The model under review builds one solid part; all positions refer to its coordinate system, in mm. A direction names the side the tool comes from. Coordinates: 2 decimals unless noted, no trailing zeros. Order: outer loops, then holes, each group sorted by start corner. A loop starts at its lowest first (then second) coordinate and runs counter-clockwise, first axis right, second up. Notation, with made-up numbers: (-4.5, 81) -> (54.5, 81) arc R24 cw to (54.5, 105) -> close; hole circle Ø2 at (-17.5, -23). An arc over 180 degrees is marked (long way). Use one line per item in the form item = value. Start each with the question number.
(1) Insertion check: pin 1 Ø6 at (y, z) = (-2.5, 21) entering from +X; pin 2 Ø5 at (y, z) = (-10.5, -10.5) entering from -X; pin 3 Ø0.7 at (x, y) = (-26, -35.5) entering from -Z. Each pin has a flat end and moves straight along its axis. Give the tip position at first contact, or say it passes through.
(2) For faces 1 (the flat face through (-27.845, -1.373, -0.571)), 2 (the flat face through (-4.2, 34.2, -25.1)), 3 (the flat face through (27.508, 35, 0)), list the 3-axis set-ups (+Z, -Z, +X, -X, +Y, -Y) from which the entire face can be reached by the end or side of a thin tool; tool diameter is ignored.
(3) Take a section at D-D (x = -21.5). State the section outline as (y, z) points.
(4) Mouldability with a two-part tool opening along Z and no side actions: class faces 4 (the cylindrical face through (0.53, -35.32, 25.17)), 5 (the flat face through (-28, 15.638, -1)), 6 (the flat face through (-27.84, 19.74, -0.79)) as +Z half, -Z half, draft (parallel to the pull), parting line (faces both ways), or undercut.
(5) Take a section at C-C (y = 0). State the section outline as (x, z) points, then the cut area to 3 significant figures.
(6) Wall thickness on line 1 along X through (y, z) = (37, 0); line 2 along Z through (x, y) = (-3.5, 25); line 3 along X through (y, z) = (14, 18): over which ranges is each line inside the solid? List them lowest first.
(7) Take a section at A-A (x = 0). State the section outline as (y, z) points (3 decimals).
(8) Take a section at B-B (z = 15). State the section outline as (x, y) points (1 decimal), then the cut area to 3 significant figures.
```python
from build123d import *

# Parameters (mm, degrees)
EXTRUDE_11_REACH             = 60.31
EXTRUDE_11_DIRECTION_2_REACH = 60.31
CUT_EXTRUDE_1_DEPTH          = 7.5
CUT_EXTRUDE_1_DEPTH_BACK     = 7.5
CUT_EXTRUDE_2_DEPTH          = 5
CUT_EXTRUDE_START            = 28.688718626
CUT_EXTRUDE_3_DEPTH          = 1.311276176
CUT_EXTRUDE_4_DEPTH          = 50
CUT_EXTRUDE_4_DEPTH_BACK     = 50
SKETCH_14_W                  = 57.911656858
SKETCH_14_H                  = 3.2
SCALE_1_SCALE                = 0.95
SKETCH_15_R                  = 3
CUT_EXTRUDE_5_DEPTH          = 56.394043173
CUT_EXTRUDE_8_DEPTH          = 56.394043173


# Read off the part's stored shape, not the designer's step: 切除-拉伸3
with BuildPart() as part:
    # 草图1 → 旋转1 (revolve)
    with BuildSketch(Plane.XY, mode=Mode.PRIVATE) as revolve_1_sk:
        Polygon((26.5, 38.4), (26.5, 36), (29, 36), (29, 0), (30, 0), (30, 40), (29, 40), (29, 38.4), align=None)
    revolve_1 = revolve(revolve_1_sk.sketch.rotate(Axis((0, 66, 0), (0, -1, 0)), 90), axis=Axis((0, 66, 0), (0, -1, 0)))

    # 镜向1: 旋转1 across plane
    add(revolve_1.mirror(Plane.ZX))

    # 凸台-拉伸11: up to this face of the body (flat: up to its plane)
    extrude_11_end = Plane(part.part.faces().sort_by_distance((0, 36, -27.320243866))[0])
    # 草图11 → 凸台-拉伸11 (add, up to the picked face)
    with BuildSketch(Plane(origin=(0, 0, 0), x_dir=(1, 0, 0), z_dir=(0, 1, 0)), mode=Mode.PRIVATE) as extrude_11_sk1:
        with BuildLine():
            Line((-13.076696831, -27), (13.076696831, -27))
            ThreePointArc((13.076696831, -27), (0, -30), (-13.076696831, -27))
        make_face()
    extrude_11_tool1 = split(extrude(extrude_11_sk1.sketch, amount=EXTRUDE_11_REACH, mode=Mode.PRIVATE), bisect_by=extrude_11_end, keep=Keep.BOTH, mode=Mode.PRIVATE)
    add(extrude_11_tool1.solids().sort_by(Axis((0, 0, 28.205296), (0, 1, 0)))[0])

    # 凸台-拉伸11 direction 2: up to this face of the body (flat: up to its plane)
    extrude_11_direction_2_end = Plane(part.part.faces().sort_by_distance((0, -36, -27.320243866))[0])
    # 草图11 → 凸台-拉伸11 direction 2 (add, up to the picked face)
    with BuildSketch(Plane(origin=(0, 0, 0), x_dir=(1, 0, 0), z_dir=(0, 1, 0)), mode=Mode.PRIVATE) as extrude_11_direction_2_sk1:
        with BuildLine():
            Line((-13.076696831, -27), (13.076696831, -27))
            ThreePointArc((13.076696831, -27), (0, -30), (-13.076696831, -27))
        make_face()
    extrude_11_direction_2_tool1 = split(extrude(extrude_11_direction_2_sk1.sketch, amount=-EXTRUDE_11_DIRECTION_2_REACH, mode=Mode.PRIVATE), bisect_by=extrude_11_direction_2_end, keep=Keep.BOTH, mode=Mode.PRIVATE)
    add(extrude_11_direction_2_tool1.solids().sort_by(Axis((0, 0, 28.205296), (0, -1, 0)))[0])

    # 草图12 → 切除-拉伸1 (cut, two sides: drawn at the far end of the back side and taken through both)
    with BuildSketch(Plane(origin=(0, 0, 0), x_dir=(1, 0, 0), z_dir=(0, 1, 0)).offset(-CUT_EXTRUDE_1_DEPTH_BACK)):
        with BuildLine():
            Line((0, 0), (22.520337054, 22.934948885))
            ThreePointArc((22.520337054, 22.934948885), (31.296937417, -7.32660697), (10, -30.547953473))
            Line((10, -30.547953473), (0, 0))
        make_face()
    extrude(amount=CUT_EXTRUDE_1_DEPTH + CUT_EXTRUDE_1_DEPTH_BACK, mode=Mode.SUBTRACT)

    # Sketch 3D_2 → 切除-拉伸2 (cut)
    with BuildSketch(Plane(origin=(35, 15, -4.993961669), x_dir=(-0.989973390659655, 0, 0.1412539761770484), z_dir=(0, 1, 0))):
        with BuildLine():
            Line((0, 0), (35.354485616, 0))
            Line((35.354485616, 0), (0.330334968, 4.976372773))
            ThreePointArc((0.330334968, 4.976372773), (0.075684949, 2.494126297), (0, 0))
        make_face()
    cut_extrude_2 = extrude(amount=CUT_EXTRUDE_2_DEPTH, mode=Mode.SUBTRACT)

    # 镜向2: 切除-拉伸2 across plane
    add(cut_extrude_2.mirror(Plane.ZX), mode=Mode.SUBTRACT)

    # 切除-拉伸3 outline → 切除-拉伸3 (cut)
    with BuildSketch(Plane.YZ.offset(CUT_EXTRUDE_START)):
        with BuildLine():
            Line((15, -4.237619285), (15, -0.017659399))
            add(Edge.make_bspline(
                [(15, -0.017659399), (12.884666816, -0.017659399), (12.884666816, -2.127639342), (12.884666816, -4.237619285), (15, -4.237619285)],
                knots=[3.141592654, 3.141592654, 3.141592654, 4.71238898, 4.71238898, 6.283185307, 6.283185307, 6.283185307], degree=2, weights=[1, 0.707106781, 1, 0.707106781, 1]))
        make_face()
    cut_extrude_3 = extrude(amount=CUT_EXTRUDE_3_DEPTH, mode=Mode.SUBTRACT)

    # 镜向3: 切除-拉伸3 across plane
    add(cut_extrude_3.mirror(Plane.ZX), mode=Mode.SUBTRACT)

    # 草图14 → 切除-拉伸4 (cut, two sides: drawn at the far end of the back side and taken through both)
    with BuildSketch(Plane(origin=(0, 0, 0), x_dir=(1, 0, 0), z_dir=(0, 1, 0)).offset(-CUT_EXTRUDE_4_DEPTH_BACK)):
        Rectangle(SKETCH_14_W, SKETCH_14_H)
    extrude(amount=CUT_EXTRUDE_4_DEPTH + CUT_EXTRUDE_4_DEPTH_BACK, mode=Mode.SUBTRACT)


with BuildPart() as part_1:
    # 缩放比例1: scaled about (0, 0, 0)
    add(part.part.scale(SCALE_1_SCALE))

    # 草图15 → 切除-拉伸5 (cut, through all)
    with BuildSketch(Plane.XY):
        Circle(SKETCH_15_R)
    extrude(amount=-CUT_EXTRUDE_5_DEPTH, mode=Mode.SUBTRACT)

    # 草图17 → 切除-拉伸8 (cut, through all)
    with BuildSketch(Plane(origin=(0, 0, 0), x_dir=(0, 0, -1), z_dir=(1, 0, 0))):
        Polygon((-7.160216771, -7.13563981), (-7.160216771, -3.80592806), (8.522673115, 1.128292258), (-7.160216771, 5.828299564), (-7.160216771, 8.761718002), (11.264359726, 3.240054279), (11.264359726, -1.338817901), align=None)
        Polygon((-7.160216771, 13.060987956), (-7.160216771, 15.637647282), (8.522673115, 15.637647282), (-7.160216771, 23.954695298), (-7.160216771, 26.120129901), (11.264359726, 26.120129901), (11.264359726, 23.954695298), (-3.480090007, 23.954695298), (11.264359726, 16.13532672), (11.264359726, 13.060987956), align=None)
        Polygon((11.264359726, -11.172137384), (11.264359726, -24.820978501), (8.522673115, -24.820978501), (8.522673115, -15.337987323), (-7.160216771, -24.820978501), (-7.160216771, -11.172137384), (-4.532843234, -11.172137384), (-4.532843234, -20.724250381), align=None)
    extrude(amount=-CUT_EXTRUDE_8_DEPTH, mode=Mode.SUBTRACT)


solid = part_1.part
```
Findings:
q1.pin_1 = -13.53
q1.pin_2 = -27.35
q1.pin_3 = -12.42
q2.face_1 = +X, -X
q2.face_2 = none
q2.face_3 = +Y, -Y
q3.outline = (-38, -18.71) -> (38, -18.71) -> (38, -17.23) -> (36.48, -17.23) -> (36.48, -13.1) -> (34.2, -13.1) -> (34.2, -17.23) -> (-34.2, -17.23) -> (-34.2, -13.1) -> (-36.48, -13.1) -> (-36.48, -17.23) -> (-38, -17.23) -> close; (-38, 17.23) -> (-36.48, 17.23) -> (-36.48, 13.1) -> (-34.2, 13.1) -> (-34.2, 17.23) -> (34.2, 17.23) -> (34.2, 13.1) -> (36.48, 13.1) -> (36.48, 17.23) -> (38, 17.23) -> (38, 18.71) -> (-38, 18.71) -> close
q4.face_4 = undercut
q4.face_5 = draft
q4.face_6 = undercut
q5.outline = (-28.07, -4.94) -> (-27.1, -4.94) arc R27.55 cw to (-10.05, 25.65) -> (8.4, 25.65) -> (8.87, 27.09) arc R28.5 ccw to start; (-26.18, -11.26) arc R28.5 ccw to (-3, -28.34) -> (-3, -27.39) arc R27.55 cw to (-25.14, -11.26) -> close; (3, -28.34) arc R28.5 ccw to (19.97, -20.34) -> (19.3, -19.66) arc R27.55 cw to (3, -27.39) -> close
q5.area = 126 mm²
q6.line_1 = -28.5 to -27.55, 27.55 to 28.5
q6.line_2 = -28.28 to -27.33, 25.65 to 28.28
q6.line_3 = -22.1 to -20.86, 20.86 to 22.1
q7.outline = (-38, -28.5) -> (-3, -28.5) -> (-3, -27.55) -> (-34.2, -27.55) -> (-34.2, -25.175) -> (-36.48, -25.175) -> (-36.48, -27.55) -> (-38, -27.55) -> close; (-38, 27.55) -> (-36.48, 27.55) -> (-36.48, 25.175) -> (-34.2, 25.175) -> (-34.2, 25.65) -> (34.2, 25.65) -> (34.2, 25.175) -> (36.48, 25.175) -> (36.48, 27.55) -> (38, 27.55) -> (38, 28.5) -> (-38, 28.5) -> close; (3, -28.5) -> (38, -28.5) -> (38, -27.55) -> (36.48, -27.55) -> (36.48, -25.175) -> (34.2, -25.175) -> (34.2, -27.55) -> (3, -27.55) -> close
q8.outline = (-24.2, -38) -> (-23.1, -38) -> (-23.1, -36.5) -> (-20.2, -36.5) -> (-20.2, -34.2) -> (-23.1, -34.2) -> (-23.1, 34.2) -> (-20.2, 34.2) -> (-20.2, 36.5) -> (-23.1, 36.5) -> (-23.1, 38) -> (-24.2, 38) -> close; (20.2, -36.5) -> (23.1, -36.5) -> (23.1, -38) -> (24.2, -38) -> (24.2, -7.1) -> (23.1, -7.1) -> (23.1, -34.2) -> (20.2, -34.2) -> close; (20.2, 34.2) -> (23.1, 34.2) -> (23.1, 7.1) -> (24.2, 7.1) -> (24.2, 38) -> (23.1, 38) -> (23.1, 36.5) -> (20.2, 36.5) -> close
q8.area = 181 mm²
